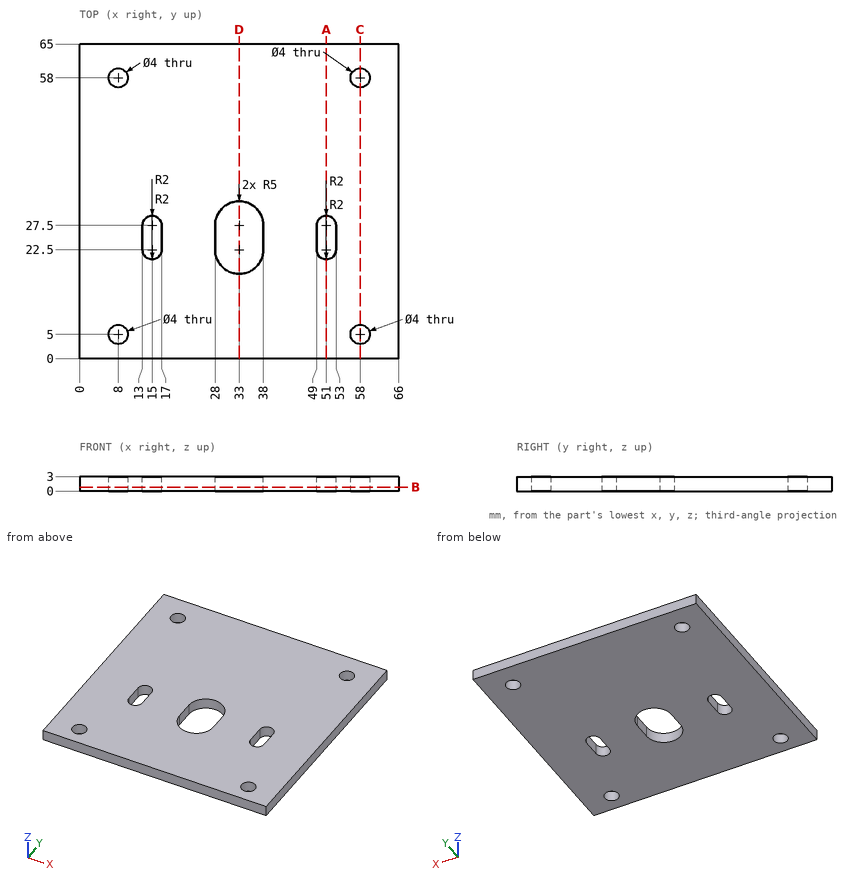
The drawing under review shows one solid part. Ordinate dimensions are in mm from its lowest x, y, z. Coordinates: 2 decimals unless noted, no trailing zeros. Loops run counter-clockwise (first coordinate to the right, second up) from the corner with the lowest first, then second, coordinate; pieces in that order, holes last.
Item 1: Wall thickness on L1, parallel to Y at x = 58, z = 1.5; L2, parallel to Y at x = 8.5, z = 2.3; L3, parallel to Y at x = 36, z = 1.8: over which ranges is each line inside the solid? List them lowest first.
Completed:
L1: y = 0 to 3, 7 to 56, 60 to 65
L2: y = 0 to 3.06, 6.94 to 56.06, 59.94 to 65
L3: y = 0 to 18.5, 31.5 to 65
Item 2: Add section A-A (x = 51). Write out the cut boundary in (y, z), and give its area (3 significant figures).
Completed:
outline: (0, 0) - (20.5, 0) - (20.5, 3) - (0, 3) - close; (29.5, 0) - (65, 0) - (65, 3) - (29.5, 3) - close
area: 168 mm2
Item 3: Add section B-B (z = 0.8). Write out the cut boundary in (x, y).
Completed:
outline: (0, 0) - (66, 0) - (66, 65) - (0, 65) - close; hole circle Ø4 at (8, 5); hole circle Ø4 at (8, 58); hole (13, 22.5) arc R2 ccw to (17, 22.5) - (17, 27.5) arc R2 ccw to (13, 27.5) - close; hole (28, 22.5) arc R5 ccw to (38, 22.5) - (38, 27.5) arc R5 ccw to (28, 27.5) - close; hole (49, 22.5) arc R2 ccw to (53, 22.5) - (53, 27.5) arc R2 ccw to (49, 27.5) - close; hole circle Ø4 at (58, 5); hole circle Ø4 at (58, 58)
Item 4: Add section D-D (x = 33). Write out the cut boundary in (y, z).
Completed:
outline: (0, 0) - (17.5, 0) - (17.5, 3) - (0, 3) - close; (32.5, 0) - (65, 0) - (65, 3) - (32.5, 3) - close
Item 5: Add section C-C (x = 58). Write out the cut boundary in (y, z).
Completed:
outline: (0, 0) - (3, 0) - (3, 3) - (0, 3) - close; (7, 0) - (56, 0) - (56, 3) - (7, 3) - close; (60, 0) - (65, 0) - (65, 3) - (60, 3) - close
